Design review of the part built by this model. Coordinates are the model's own, in mm. A direction names the side the tool comes from. Give positions to 0.01 mm unless a question says otherwise; leave off trailing zeros. Write each loop counter-clockwise with the first axis right and the second up, starting at its lowest first coordinate (ties: lowest second). Pieces come first, ordered by that corner, then holes. Notation, with made-up numbers: M 34.25,-5 L 73.25,-5 A31 ccw 73.25,34 Z; hole C -25,-16.5 d10. An arc over 180 degrees is marked long. Use a Markdown table: item, result. Add a question column.
Autodesk Inventor part; units mm, degrees
ref_plane "Work Plane1" through (0, 0, 2.54) normal (0, 0, 1) x (1, 0, 0)
ref_plane "YZ Plane" through (0, 0, 0) normal (1, 0, 0) x (0, 1, 0)
ref_plane "XZ Plane" through (0, 0, 0) normal (0, 1, 0) x (-1, 0, 0)
ref_plane "Work Plane1" through (0, 0, 2.54) normal (0, 0, 1) x (1, 0, 0)
sketch "Sketch2" plane through (0, 0, 2.54) normal (0, 0, 1) x (1, 0, 0)
  line L0 (6.5, -32.5) -> (6.5, -38.5)
  line L1 (6.5, -38.5) -> (0.5, -38.5)
  line L2 (0.5, -38.5) -> (0.5, -32.5)
  line L3 (0.5, -32.5) -> (6.5, -32.5)
  circle A0 centre (19.75, -34.75) radius 5.75
  line L4 (43.5, -29) -> (43.5, -41.5)
  line L5 (43.5, -41.5) -> (30, -41.5)
  line L6 (30, -41.5) -> (30, -29)
  line L7 (30, -29) -> (43.5, -29)
  circle A1 centre (44, 41) radius 1.5
  circle A2 centre (-44, 41) radius 1.5
  line L8 (46.5, 43.5) -> (-46.5, 43.5)
  line L9 (-46.5, 43.5) -> (-46.5, -43.5)
  line L10 (-46.5, -43.5) -> (46.5, -43.5)
  line L11 (46.5, -43.5) -> (46.5, 43.5)
  line L12 (-46.5, 43.5) -> (46.5, 43.5)
  line L13 (46.5, 43.5) -> (46.5, -26.5)
  line L14 (46.5, -26.5) -> (-46.5, -26.5)
  line L15 (-46.5, -26.5) -> (-46.5, 43.5)
  circle A3 centre (-44, 41) radius 1.5
  circle A4 centre (44, 41) radius 1.5
  circle A5 centre (44, -24) radius 1.5
  circle A6 centre (-44, -24) radius 1.5
  line L16 (-45.5, -20.479) -> (-45.5, -25.5) construction
  line L17 (-45.5, -25.5) -> (-36.292, -25.5) construction
  line L18 (45.5, -16.7483) -> (45.5, -25.5) construction
  line L19 (45.5, -25.5) -> (38.0013, -25.5) construction
  circle A7 centre (-44, -24) radius 1.5
  circle A8 centre (44, -24) radius 1.5
  point P0 (0, 0)
  dimension "d0" = 70
  dimension "d1" = 3
  dimension "d2" = 3
  dimension "d3" = 1
  dimension "d4" = 1
  dimension "d5" = 1
  dimension "d6" = 1
  dimension "d21" = 65
  dimension "d22" = 65
extrude "Tykkelsen Grøn PCB" add sketch "Sketch2" along normal blind 1.5 contours L11 L14 L9 L8
sketch "Sketch3" plane through (0, 0, 4.04) normal (0, 0, 1) x (1, 0, 0)
  line L0 (-46.5, 43.5) -> (-46.5, -26.5)
  line L1 (46.5, -26.5) -> (46.5, 43.5)
  line L2 (46.5, 43.5) -> (-46.5, 43.5)
  line L3 (-39, 34.5) -> (39, 34.5)
  line L4 (39, 34.5) -> (39, -16.5)
  line L5 (39, -16.5) -> (-39, -16.5)
  line L6 (-39, -16.5) -> (-39, 34.5)
  point P0 (0, 0)
  dimension "d9" = 51
  dimension "d10" = 78
  dimension "d11" = 7.5
  dimension "d12" = 7.5
  dimension "d13" = 9
extrude "Skærm" add sketch "Sketch3" along normal blind 8
sketch "Sketch5" plane through (0, 0, 12.04) normal (0, 0, 1) x (1, 0, 0)
  line L0 (39, 34.5) -> (-39, 34.5)
  line L1 (-39, 34.5) -> (-39, -16.5)
  line L2 (-39, -16.5) -> (39, -16.5)
  line L3 (39, -16.5) -> (39, 34.5)
  line L4 (-34.5, 28.5) -> (34.5, 28.5)
  line L5 (36.5, 26.5) -> (36.5, -8.5)
  line L6 (34.5, -10.5) -> (-34.5, -10.5)
  line L7 (-36.5, -8.5) -> (-36.5, 26.5)
  arc A0 (-34.5, 28.5) -> (-36.5, 26.5) centre (-34.5, 26.5) ccw
  arc A1 (36.5, 26.5) -> (34.5, 28.5) centre (34.5, 26.5) ccw
  arc A2 (34.5, -10.5) -> (36.5, -8.5) centre (34.5, -8.5) ccw
  arc A3 (-36.5, -8.5) -> (-34.5, -10.5) centre (-34.5, -8.5) ccw
  point P0 (0, 0)
  dimension "d23" = 2.5
  dimension "d24" = 6
  dimension "d25" = 2.5
  dimension "d26" = 6
  dimension "d27" = 2
extrude "Hul ned i skærm" cut sketch "Sketch5" against normal blind 0.7 contours L4 A1 L5 A2 L6 A3 L7 A0
sketch "Sketch4" plane through (0, 0, 4.04) normal (0, 0, 1) x (1, 0, 0)
  line L0 (-39, -16.5) -> (-39, 34.5)
  line L1 (-39, 34.5) -> (39, 34.5)
  line L2 (-45.5, 30.5) -> (-39, 30.5)
  line L3 (-39, 30.5) -> (-39, -11.5)
  line L4 (-39, -11.5) -> (-45.5, -11.5)
  line L5 (-45.5, -11.5) -> (-45.5, 30.5)
  point P0 (0, 0)
  dimension "d16" = 42
  dimension "d17" = 6.5
  dimension "d18" = 4
extrude "Hvid ting" add sketch "Sketch4" along normal blind 3.5
equation "\"d11\" = d12"
properties part number "Grøn PCB"
(1) Add section A-A on y = 41. Give the boundary of the cut face in (x, z), then the cut area to 4 significant figures.
(2) Add section C-C on x = 29. Give the boundary of the cut face in (y, z), then the cut area to 3 significant figures.
(3) Add section D-D on z = 5.25. Give the boundary of the cut face in (x, y), then the cut area to 3 significant figures.
(4) Wall thickness on L1, parallel to Y at x = 44, z = 3.05; L2, parallel to Y at x = 43, z = 3.75; L3, parallel to Z at x = -1.5, y = -2.5: over which ranges is each line inside the solid? List them lowest first.
(5) Machinability: for faces 1 (the flat face through (-42, -11.5, 6)), 2 (the flat face through (-45.5, 9, 6)), 3 (the flat face through (1, -16.5, 8)), 4 (the cylindrical face through (-35.9, 27.93, 11.69)), which of the approach directions +Z, -Z, +X, -X, +Y, -Y give a long, thin tool a straight path to every point of the face, cutting with its end or side? Answer none if there is none.
(6) Add section B-B on y = -1.5. Give the boundary of the cut face in (x, z).
(7) For pin 1 (2 mm diameter, centred on y = 24, z = 8, fed in from +X); pin 2 (3 mm diameter, centred on x = 0, y = -19, fed in from +Z); pin 3 (0.6 mm diameter, centred on x = -0.5, z = 11.5, fed in from +Y), all flat-tipped, find the tip position at first contact; note any pin that passes through.
(8) The part is to be moulded in two halves that separate along Y. For faces 5 (the flat face through (-1, 34.5, 8)), 6 (the flat face through (-1, 9, 11.34)), 7 (the flat face through (-42, 10, 7.54)), say which applies: released by +Y, released by -Y, zero draft, split by the parting line, or undercut.
From the geometry:
| question | item | result |
|---|---|---|
| 1 | outline | M -46.5,2.54 L -45.5,2.54 L -45.5,4.04 L -46.5,4.04 Z; M -42.5,2.54 L 42.5,2.54 L 42.5,4.04 L -42.5,4.04 Z; M 45.5,2.54 L 46.5,2.54 L 46.5,4.04 L 45.5,4.04 Z |
| 1 | area | 130.5 mm^2 |
| 2 | outline | M -26.5,2.54 L 43.5,2.54 L 43.5,4.04 L 34.5,4.04 L 34.5,12.04 L 28.5,12.04 L 28.5,11.34 L -10.5,11.34 L -10.5,12.04 L -16.5,12.04 L -16.5,4.04 L -26.5,4.04 Z |
| 2 | area | 486 mm^2 |
| 3 | outline | M -45.5,-11.5 L -39,-11.5 L -39,-16.5 L 39,-16.5 L 39,34.5 L -39,34.5 L -39,30.5 L -45.5,30.5 Z |
| 3 | area | 4,250 mm^2 |
| 4 | L1 | y = -26.5 to -25.5, -22.5 to 39.5, 42.5 to 43.5 |
| 4 | L2 | y = -26.5 to -25.12, -22.88 to 39.88, 42.12 to 43.5 |
| 4 | L3 | z = 2.54 to 11.34 |
| 5 | face 1 | +Z, -X, -Y |
| 5 | face 2 | +Z, -X, +Y, -Y |
| 5 | face 3 | +Z, +X, -X, -Y |
| 5 | face 4 | +Z |
| 6 | outline | M -46.5,2.54 L 46.5,2.54 L 46.5,4.04 L 39,4.04 L 39,12.04 L 36.5,12.04 L 36.5,11.34 L -36.5,11.34 L -36.5,12.04 L -39,12.04 L -39,7.54 L -45.5,7.54 L -45.5,4.04 L -46.5,4.04 Z |
| 7 | pin 1 | stops at x = 39 |
| 7 | pin 2 | stops at z = 4.04 |
| 7 | pin 3 | stops at y = 34.5 |
| 8 | face 5 | released by +Y |
| 8 | face 6 | undercut |
| 8 | face 7 | zero draft |
